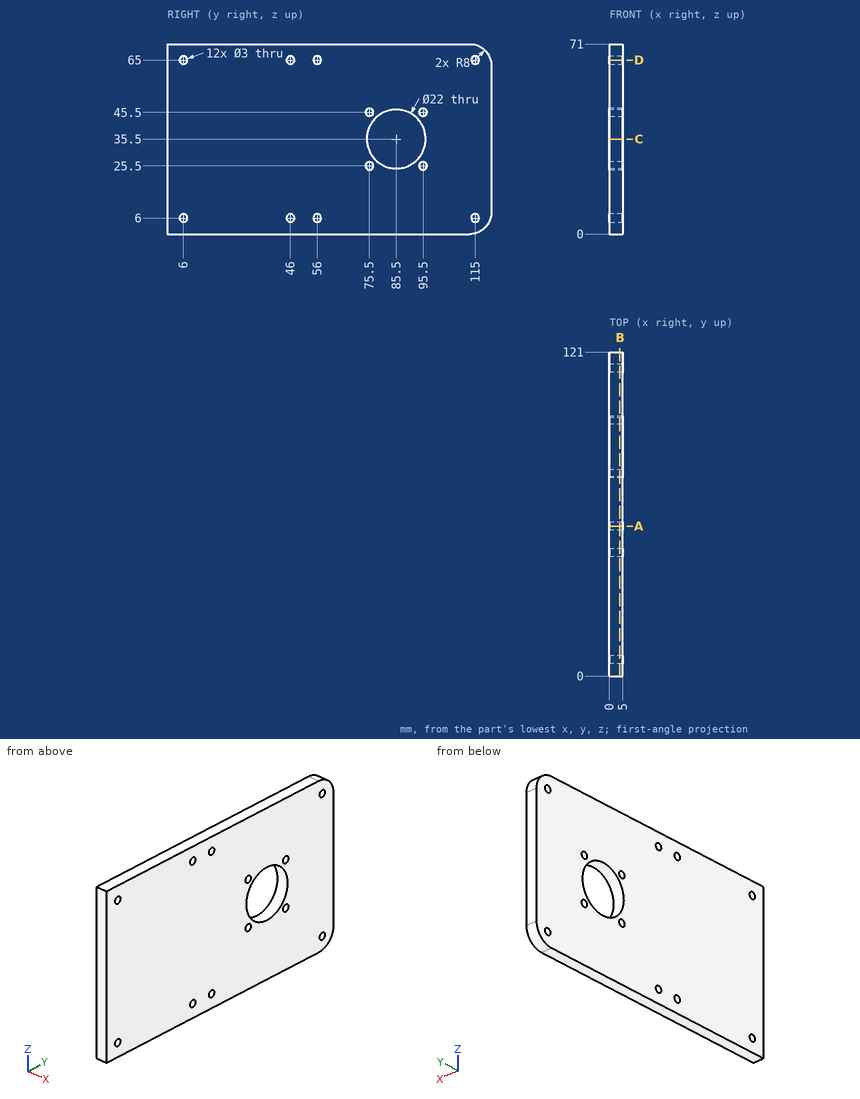
Study the drawing (mm; zero at the part's minimum x, y, z) and answer. Give positions to 0.01 mm unless a question says otherwise; leave off trailing zeros. Write each loop counter-clockwise with the first axis right and the second up, starting at its lowest first coordinate (ties: lowest second). Pieces come first, ordered by that corner, then holes. Notation, with made-up numbers: (-4, 71.25) - (24, 71.25) arc R14 cw to (24, 94.25) - close; hole circle Ø7 at (16.25, 89.25). An arc over 180 degrees is marked (long way). Write item = value, one per line. Start each with the question number.
Item 1: Find section A-A (y = 56). Give the vertices of the cut face in (x, z), then the cut area to 3 significant figures.
Item 2: Find section B-B (x = 3.95). State how many separate pieces and enclosed holes the cut face has, then the cut area to 3 significant figures.
Item 3: Find section C-C (z = 35.5). Give the vertices of the cut face in (x, y).
Item 4: Find section D-D (z = 65). Give the vertices of the cut face in (x, y), then the cut area to 3 significant figures.
Item 5: This flat-tipped pin is pushed along its axis until it touches: P1, Ø2.5, axis at y = 56, z = 6, coming from the +X side. Where does it stop, or does it pass through?
Item 6: Find the intervals of material crossed by probe 1 along Y at (x, z) = (1.95, 65); probe 2 along Z at (x, y) = (2.75, 75.5); probe 3 along Z at (x, y) = (4.6, 55), in increasing order. Write a range as [from, to].
Response:
q1.outline = (0, 0) - (5, 0) - (5, 4.5) - (0, 4.5) - close; (0, 7.5) - (5, 7.5) - (5, 63.5) - (0, 63.5) - close; (0, 66.5) - (5, 66.5) - (5, 71) - (0, 71) - close
q1.area = 325 mm²
q2.separate_pieces = 1
q2.enclosed_holes = 13
q2.area = 8,100 mm²
q3.outline = (0, 0) - (5, 0) - (5, 74.5) - (0, 74.5) - close; (0, 96.5) - (5, 96.5) - (5, 121) - (0, 121) - close
q4.outline = (0, 0) - (5, 0) - (5, 4.5) - (0, 4.5) - close; (0, 7.5) - (5, 7.5) - (5, 44.5) - (0, 44.5) - close; (0, 47.5) - (5, 47.5) - (5, 54.5) - (0, 54.5) - close; (0, 57.5) - (5, 57.5) - (5, 113.5) - (0, 113.5) - close; (0, 116.5) - (5, 116.5) - (5, 120.75) - (0, 120.75) - close
q4.area = 544 mm²
q5.P1 = through
q6.probe_1 = [0, 4.5], [7.5, 44.5], [47.5, 54.5], [57.5, 113.5], [116.5, 120.75]
q6.probe_2 = [0, 24], [27, 30.92], [40.08, 44], [47, 71]
q6.probe_3 = [0, 4.88], [7.12, 63.88], [66.12, 71]
